Could you check a few things on this model? Use its own coordinates, in mm. Face numbers are marked on the shaded views. A direction names the side the tool comes from. Coordinates: 2 decimals unless noted, no trailing zeros. Write each loop counter-clockwise with the first axis right and the second up, starting at its lowest first coordinate (ties: lowest second). Pieces come first, ordered by that corner, then holes. Notation, with made-up numbers: M 64,35.5 L 112,35.5 A28 cw 112,71.5 Z; hole C 26,77.25 d1. An arc over 180 degrees is marked long. Write item = value, one per line.
```python
from build123d import *

# Parameters (mm, degrees)
F0_R         = 11
F0_R_2       = 1.5
F1_DEPTH     = 10
F3_DEPTH     = 25
F4_T4_DEPTH  = 31.4403610405
F4_S5_R      = 9
F4_T6_DEPTH  = 17
F4_T10_DEPTH = 33.7217724143
F4_S11_R     = 7
F4_T12_DEPTH = 19
F4_T16_DEPTH = 39.2279914145
F4_S17_R     = 5
F4_T18_DEPTH = 21


# Not quite as in the source:
# - a fillet or chamfer that OpenCascade refuses, or shapes differently, is made with other operations: its cross-section is extruded or revolved along the edge and cut away or added


with BuildPart() as f1:
    # F0 (on Top) → F1 (new body)
    with BuildSketch(Plane.XY):
        Circle(F0_R)
        Circle(F0_R_2, mode=Mode.SUBTRACT)
    extrude(amount=F1_DEPTH)

    # F2 (on face) → F3 (cut)
    with BuildSketch(Plane(origin=(0, 0, 0), x_dir=(1, 0, 0), z_dir=(0, 0, -1))):
        with BuildLine():
            ThreePointArc((0, -9), (-6.3639610307, -6.3639610307), (-9, 0))
            Line((-9, 0), (-11, 0))
            ThreePointArc((-11, 0), (-7.7781745931, -7.7781745931), (0, -11))
            Line((0, -11), (0, -9))
        make_face()
        with BuildLine():
            Line((11, 0), (9, 0))
            ThreePointArc((9, 0), (6.3639610307, -6.3639610307), (0, -9))
            Line((0, -9), (0, -11))
            ThreePointArc((0, -11), (7.7781745931, -7.7781745931), (11, 0))
        make_face()
        with BuildLine():
            Line((9, 0), (7, 0))
            ThreePointArc((7, 0), (4.9497474683, -4.9497474683), (0, -7))
            Line((0, -7), (0, -9))
            ThreePointArc((0, -9), (6.3639610307, -6.3639610307), (9, 0))
        make_face()
        with BuildLine():
            Line((0, 7), (0, 5))
            ThreePointArc((0, 5), (3.5355339059, 3.5355339059), (5, 0))
            Line((5, 0), (7, 0))
            ThreePointArc((7, 0), (4.9497474683, 4.9497474683), (0, 7))
        make_face()
        with BuildLine():
            Line((0, 9), (0, 7))
            ThreePointArc((0, 7), (4.9497474683, 4.9497474683), (7, 0))
            Line((7, 0), (9, 0))
            ThreePointArc((9, 0), (6.3639610307, 6.3639610307), (0, 9))
        make_face()
        with BuildLine():
            Line((0, 11), (0, 9))
            ThreePointArc((0, 9), (6.3639610307, 6.3639610307), (9, 0))
            Line((9, 0), (11, 0))
            ThreePointArc((11, 0), (7.7781745931, 7.7781745931), (0, 11))
        make_face()
    extrude(amount=-F3_DEPTH, mode=Mode.SUBTRACT)

    # F4: chamfer of 3 on 3 edges, made by hand


with BuildPart() as f4_tool2:
    # F4_s3 → F4_t4 (new body)
    with BuildSketch(Plane.XY.offset(-10.7201805202)):
        with BuildLine():
            Line((-10.1972729198, -4.125), (-7.4161984871, 0))
            Line((-7.4161984871, 0), (-11, 0))
            ThreePointArc((-11, 0), (-10.7891469286, -2.1434338231), (-10.1972729198, -4.125))
        make_face()
    extrude(amount=F4_T4_DEPTH)

    # F4_s5 → F4_t6 (cut, symmetric)
    with BuildSketch(Plane.XY.offset(5)):
        Circle(F4_S5_R)
    extrude(amount=F4_T6_DEPTH, both=True, mode=Mode.SUBTRACT)


with BuildPart() as f1_1:
    add(f1.part)

    # F4_t1: cut F4_tool2
    add(f4_tool2.part, mode=Mode.SUBTRACT)


with BuildPart() as f4_tool8:
    # F4_s9 → F4_t10 (new body)
    with BuildSketch(Plane.XY.offset(-11.8608862072)):
        with BuildLine():
            Line((-4.5, 7.7942286341), (0, 5.1961524227))
            Line((0, 5.1961524227), (0, 9))
            ThreePointArc((0, 9), (-2.3715637944, 8.6819171367), (-4.5, 7.7942286341))
        make_face()
    extrude(amount=F4_T10_DEPTH)

    # F4_s11 → F4_t12 (cut, symmetric)
    with BuildSketch(Plane.XY.offset(5)):
        Circle(F4_S11_R)
    extrude(amount=F4_T12_DEPTH, both=True, mode=Mode.SUBTRACT)


with BuildPart() as f1_2:
    add(f1_1.part)

    # F4_t7: cut F4_tool8
    add(f4_tool8.part, mode=Mode.SUBTRACT)


with BuildPart() as f4_tool14:
    # F4_s15 → F4_t16 (new body)
    with BuildSketch(Plane.XY.offset(-14.6139957073)):
        with BuildLine():
            Line((4.6300647944, 5.25), (2.6457513111, 0))
            Line((2.6457513111, 0), (7, 0))
            ThreePointArc((7, 0), (6.3609005548, 2.9221471784), (4.6300647944, 5.25))
        make_face()
    extrude(amount=F4_T16_DEPTH)

    # F4_s17 → F4_t18 (cut, symmetric)
    with BuildSketch(Plane.XY.offset(5)):
        Circle(F4_S17_R)
    extrude(amount=F4_T18_DEPTH, both=True, mode=Mode.SUBTRACT)


with BuildPart() as f1_3:
    add(f1_2.part)

    # F4_t13: cut F4_tool14
    add(f4_tool14.part, mode=Mode.SUBTRACT)


solid = f1_3.part
```
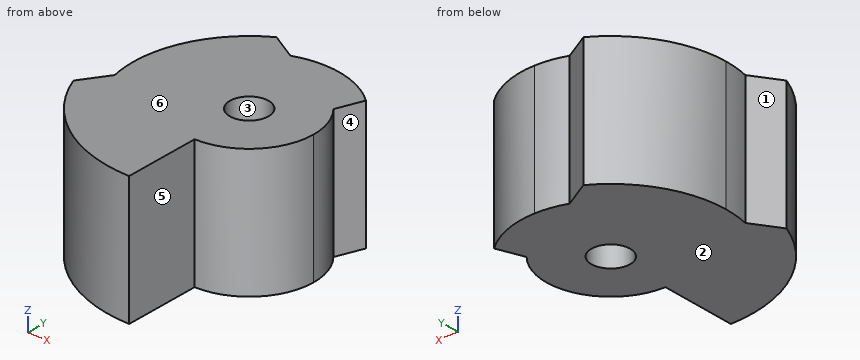
Item 1: Imagine slicing it at C-C (x = -7.25). Write out the boundary of the cut face in (y, z).
Numbers:
outline = M -8.27,0 L 5.33,0 L 5.33,10 L -8.27,10 Z
Item 2: For the marked faces 4, 5 and 6, which set-ups out of +Z, -Z, +X, -X, +Y, -Y let a thin tool reach every point of the face, with its end or its side?
Numbers:
face_4 = +Z, -Z, +X
face_5 = +Z, -Z, +X, -Y
face_6 = +Z, +X, -X, +Y, -Y
Item 3: Imagine slicing it at A-A (z = 2.75). Write out the boundary of the cut face in (x, y) (3 decimals), and give its area (3 significant figures).
Numbers:
outline = M -10.197,-4.125 A11 ccw 0,-11 L 0,-5 A5 ccw 3.851,3.189 L 4.63,5.25 A7 ccw -2.394,6.578 L -4.5,7.794 A9 ccw -8.772,-2.011 Z; hole C 0,0 d3
area = 187 mm²
Item 4: I'm going to push flat-ended pins straight in: P1, Ø1, axis at y = 1, z = 2, coming from the +X side; P2, Ø5, axis at x = -8, z = 3, coming from the -Y side; P3, Ø1, axis at y = 2, z = 7, coming from the -X side; P4, Ø5, axis at x = 0, y = 0, coming from the -Z side. Where does each tip first touch, or does it pass through?
Numbers:
P1 = 4.97
P2 = -9.53
P3 = -8.87
P4 = 0
Item 5: Imagine slicing it at B-B (y = 0.25). Write out the boundary of the cut face in (x, z), and give its area (3 significant figures).
Numbers:
outline = M -9,0 L -1.48,0 L -1.48,10 L -9,10 Z; M 1.48,0 L 4.99,0 L 4.99,10 L 1.48,10 Z
area = 110 mm²
Item 6: If I drill on line 1 along Y through (x, z) = (-1, 3.5); line 2 along Y through (x, z) = (-0.5, 9.75); line 3 along Y through (x, z) = (-8.25, 1.5), over which ranges is the centre line in solid material (lowest first)?
Numbers:
line_1 = -10.95 to -1.12, 1.12 to 6.93
line_2 = -10.99 to -1.41, 1.41 to 6.98
line_3 = -7.28 to 3.6
Item 7: Imagine slicing it at D-D (y = 3.5). Write out the boundary of the cut face in (x, z), and give its area (3 significant figures).
Numbers:
outline = M -8.29,0 L 3.97,0 L 3.97,10 L -8.29,10 Z
area = 123 mm²
Item 8: If we mould it in two halves opening along X, with no side actions, what happens to the marked faces 1, 2 and 3? For each: pulls with the +X half, pulls with the -X half, needs draft (parallel to the pull), parting line crosses it, or undercut.
Numbers:
face_1 = pulls with the -X half
face_2 = needs draft
face_3 = undercut
